from build123d import *

# Parameters (mm, degrees)
FILLET1_R           = 10
SKETCH5_R           = 0.5
BOSS_EXTRUDE1_DEPTH = 60
CUT_EXTRUDE1_START  = -5
SKETCH7_R           = 0.5
CUT_EXTRUDE1_DEPTH  = 5


with BuildPart() as part:
    # Sketch3 → Revolve1 (revolve)
    with BuildSketch(Plane.XY, mode=Mode.PRIVATE) as revolve1_sk:
        Polygon((0, 60), (0, 44.835164835), (12.405575488, 0), (16.601578962, 0), align=None)
    revolve(revolve1_sk.sketch.rotate(Axis((0, 0, 0), (0, 1, 0)), 90), axis=Axis((0, 0, 0), (0, 1, 0)))

    # Fillet1
    # the kernel refuses this fillet: 10 mm, written as the material it takes off along each edge
    with BuildSketch(Plane(origin=(0, 0, 0), x_dir=(0, 0, -1), z_dir=(1, 0, 0))) as fillet1_piece_1:
        with BuildLine():
            CenterArc((4.523166195, 6.153667503), FILLET1_R, 322.021426145, 53.44496685)
            Line((12.405575488, 0), (12.563223674, -0.12307335))
            ThreePointArc((12.563223674, -0.12307335), (14.503577225, -0.2), (16.601578962, -0.2))
            Line((16.601578962, -0.2), (16.794336369, 0.053334622))
            Line((16.794336369, 0.053334622), (14.353793971, 8.873733224))
            Line((14.353793971, 8.873733224), (14.161036564, 8.820398602))
        make_face()
    revolve(axis=Axis((0, 0, 0), (0, 1, 0)), mode=Mode.SUBTRACT)

    # Sketch5 → Boss-Extrude1 (add)
    with BuildSketch(Plane(origin=(0, 0, 0), x_dir=(1, 0, 0), z_dir=(0, 1, 0))):
        with Locations(Location((0, 0, 0), (0, 0, 90))):
            Circle(SKETCH5_R)
    extrude(amount=BOSS_EXTRUDE1_DEPTH)

    # Sketch7 → Cut-Extrude1 (cut)
    with BuildSketch(Plane(origin=(0, 60, 0), x_dir=(1, 0, 0), z_dir=(0, 1, 0)).offset(CUT_EXTRUDE1_START)):
        with Locations(Location((0, 0, 0), (0, 0, 90))):
            Circle(SKETCH7_R)
    extrude(amount=CUT_EXTRUDE1_DEPTH, mode=Mode.SUBTRACT)


solid = part.part
Geometry: final body of the model. Coordinates: model frame, mm. Round coordinates to 2 decimals unless told otherwise and drop trailing zeros. Write each loop counter-clockwise with the first axis right and the second up, starting at its lowest first coordinate (ties: lowest second). Pieces come first, ordered by that corner, then holes. Notation, with made-up numbers: M 75.5,46.25 L 84.5,46.25 A10 ccw 84.5,61.25 Z; hole C 86.5,11.25 d6. An arc over 180 degrees is marked long. Write item = value, one per line.
Item 1: Pull-direction query (X, two-part tool) for faces 1 (the face through (-4.89, 33.852, 5.332)), 2 (the face through (3.977, 21.213, 5.187)); classes: pulls with the +X half, pulls with the -X half, needs draft (parallel to the pull), parting line crosses it, or undercut.
Findings:
face_1 = parting line crosses it
face_2 = undercut
Item 2: Section query A-A on y = 15. Return loops of the section in (x, z).
Findings:
outline = C 0,0 d24.9; C 0,0 d1; hole C 0,0 d16.51
Item 3: Material intervals for line 1 along X through (y, z) = (56.7, 0); line 2 along X through (y, z) = (55.9, 0); line 3 along Z through (x, y) = (-1.25, 49), sorted ascending. Write a range as [from, to].
Findings:
line_1 = [-0.91, -0.5], [0.5, 0.91]
line_2 = [-1.13, -0.5], [0.5, 1.13]
line_3 = [-2.78, 2.78]
Item 4: Pin query (flat end, axial travel): P1, Ø0.8, axis at x = 0, z = 0, coming from the +Y side; P2, Ø3, axis at y = 14.5, z = -4, coming from the -X side; P3, Ø3, axis at x = -11, y = 33, coming from the +Z side; P4, Ø1, axis at y = 14, z = -5.5, coming from the +X side. Return the tip coordinate at first contact, or that it passes through.
Findings:
P1 = 55
P2 = -12.55
P3 = through
P4 = 11.75
